from build123d import *

# Parameters (mm, degrees)
F0_R     = 3
F0_R_2   = 2.5
F1_DEPTH = 4
F0_R_3   = 5.5
F0_R_4   = 5
F2_START = 0.2
F2_DEPTH = 3.6
F3_SIZE  = 0.1


with BuildPart() as f1:
    # F0 (on Top) → F1 (new body)
    with BuildSketch(Plane.XY):
        Circle(F0_R)
        Circle(F0_R_2, mode=Mode.SUBTRACT)
    extrude(amount=F1_DEPTH)



with BuildPart() as f1b:
    # F0 (on Top) → F1, piece 2 (new body)
    with BuildSketch(Plane.XY):
        Circle(F0_R_3)
        Circle(F0_R_4, mode=Mode.SUBTRACT)
    extrude(amount=F1_DEPTH)


with BuildPart() as f1_1:
    add(f1.part)

    add(f1b.part)  # F2 merges F1b
    # F0 (on Top) → F2 (join)
    with BuildSketch(Plane.XY.offset(F2_START)):
        Circle(F0_R_4)
        Circle(F0_R, mode=Mode.SUBTRACT)
    extrude(amount=F2_DEPTH)

    # F3
    f3_edges = [f1_1.edges().sort_by_distance(p)[0] for p in [
        (-3, 0, 0),
        (-2.5, 0, 0),
        (-5.5, 0, 4),
        (-5, 0, 4),
        (-3, 0, 4),
        (-2.5, 0, 4),
        (-5.5, 0, 0),
        (-5, 0, 0),
    ]]
    chamfer(f3_edges, length=F3_SIZE)


solid = f1_1.part
Source: CAD feature listing. Evaluate the final solid. Frame: model axes, mm. A direction names the side the tool comes from. Coordinates: 2 decimals unless noted, no trailing zeros. Order: outer loops, then holes, each group sorted by start corner. A loop starts at its lowest first (then second) coordinate and runs counter-clockwise, first axis right, second up. Notation, with made-up numbers: M 26.5,26 L 83.5,26 A14 ccw 83.5,46 Z; hole C -16.75,65.25 d9. An arc over 180 degrees is marked long. Write each question's results on one line, items separated by ' | '. Start each with the question number.
1. Pin query (flat end, axial travel): pin 1 (4 mm diameter, centred on x = 0, y = 0, fed in from +Z); pin 2 (2 mm diameter, centred on x = -2.5, z = 3, fed in from -Y); pin 3 (2 mm diameter, centred on y = 4.5, z = 1.5, fed in from +X); pin 4 (2 mm diameter, centred on x = 2.5, z = 2.5, fed in from +Y). Return the tip coordinate at first contact, or that it passes through.
2. Draft query along X for faces 3 (the face through (-0.1, -3.3, 0.2)), 4 (the face through (-1.19, -5.37, 1.97)). Return one class per face: +X half, -X half, draft (parallel to the pull), parting line (faces both ways), or undercut.
3. Section A-A, the plane z = 2.75. Return the cut outline in (x, y).
4. Reachability of faces 1 (the face through (-0.1, -3.3, 3.8)), 2 (the face through (-0.54, -2.44, 1.97)) from +Z, -Z, +X, -X, +Y, -Y: full face, straight path, thin tool, end or side. Return the list, or none.
5. Material intervals for L1, parallel to Y at x = 0, z = 3.7; L2, parallel to Z at x = 2, y = -4.5; L3, parallel to Y at x = -1, z = 2.7, sorted ascending.
Solution:
1) pin 1: through | pin 2: y = -5.29 | pin 3: x = 4.24 | pin 4: y = 5.29
2) face 3: undercut | face 4: parting line
3) outline: C 0,0 d11; hole C 0,0 d5
4) face 1: +Z | face 2: +Z, -Z
5) L1: -5.5 to -2.5, 2.5 to 5.5 | L2: 0.2 to 3.8 | L3: -5.41 to -2.29, 2.29 to 5.41
